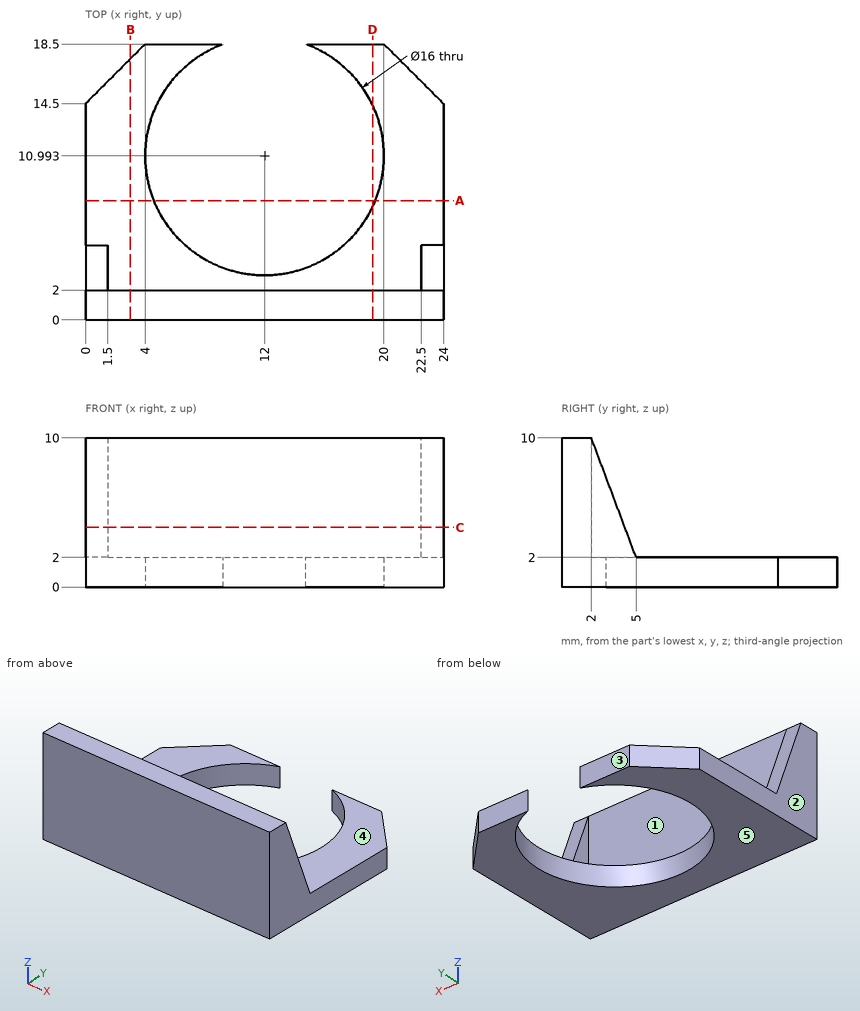
Geometry: see drawing. Coordinates: mm, zero at the bounding-box minimum. A direction names the side the tool comes from. Give positions to 0.01 mm unless a question says otherwise; leave off trailing zeros. Loops run counter-clockwise (first coordinate to the right, second up) from the corner with the lowest first, then second, coordinate; pieces in that order, holes last. Notation, with made-up numbers: (51, 46) - (102, 46) arc R14 cw to (102, 55) - close; hole circle Ø9 at (56.5, 89). An arc over 180 degrees is marked (long way). Use CSV: the item, a comma, the result in double quotes. Start each with the question number.
1. Section D-D (x = 19.25). Output: boundary loops of the cut face in (y, z) (1 decimal), then the cut area to 3 significant figures.
2. Draft query along Z for the marked faces 3, 4 and 5. Return one class per face: +Z half, -Z half, draft (parallel to the pull), parting line (faces both ways), or undercut.
3. Section C-C (z = 4). Output: boundary loops of the cut face in (x, y).
4. Section A-A (y = 8). Output: boundary loops of the cut face in (x, z), then the cut area to 3 significant figures.
5. Section B-B (x = 3). Output: boundary loops of the cut face in (y, z).
6. Pin query (flat end, axial travel): pin 1 (5 mm diameter, centred on x = 19, y = 9, fed in from +Z). Return the tip coordinate at first contact, or that it passes through.
7. Ray query, L1, parallel to X at y = 10.75, z = 1; L2, parallel to X at y = 4, z = 2.25; L3, parallel to Y at x = 20, z = 6.25. Return the intervals inside material, ascending.
8. Reachability of the marked faces 1 and 2 from +Z, -Z, +X, -X, +Y, -Y: full face, straight path, thin tool, end or side. Return the list, or none.
Response:
1,outline,"(0, 0) - (7.6, 0) - (7.6, 2) - (2, 2) - (2, 10) - (0, 10) - close; (14.4, 0) - (18.5, 0) - (18.5, 2) - (14.4, 2) - close"
1,area,"39.5 mm²"
2,face 3,"draft"
2,face 4,"+Z half"
2,face 5,"-Z half"
3,outline,"(0, 0) - (24, 0) - (24, 4.25) - (22.5, 4.25) - (22.5, 2) - (1.5, 2) - (1.5, 4.25) - (0, 4.25) - close"
4,outline,"(0, 0) - (4.58, 0) - (4.58, 2) - (0, 2) - close; (19.42, 0) - (24, 0) - (24, 2) - (19.42, 2) - close"
4,area,"18.3 mm²"
5,outline,"(0, 0) - (17.5, 0) - (17.5, 2) - (2, 2) - (2, 10) - (0, 10) - close"
6,pin 1,"z = 2"
7,L1,"0 to 4, 20 to 24"
7,L2,"0 to 1.5, 22.5 to 24"
7,L3,"0 to 2"
8,face 1,"+Z, +Y"
8,face 2,"+Z, -Z, -X, +Y, -Y"
